```python
from build123d import *

# Parameters (mm, degrees)
F1_DEPTH = 27.4
F3_DEPTH = 10
F5_DEPTH = 88.2
F6_R     = 3.700156
F7_DEPTH = 27.768068


with BuildPart() as f1:
    # F0 (on Front) → F1 (new body, symmetric)
    with BuildSketch(Plane.XZ):
        Polygon((-10.816675, 0), (0, 0), (0, 27.767068), (-52.702516, 27.767068), (-52.702516, 10.254359), (-10.816675, 10.254359), align=None)
        Polygon((0, 27.767068), (0, 0), (10.816675, 0), (54.839961, 0), align=None)
    extrude(amount=F1_DEPTH, both=True)

    # F2 (on face) → F3 (cut)
    with BuildSketch(Plane.XZ.offset(27.4)):
        Polygon((10.816675, 22.290271), (10.816675, 0), (54.839961, 0), align=None)
    extrude(amount=-F3_DEPTH, mode=Mode.SUBTRACT)

    # F4 (on Right) → F5 (cut, symmetric)
    with BuildSketch(Plane.YZ):
        Polygon((-4.211452, 25.516083), (0, 25.516083), (4.211452, 25.516083), (4.211452, 28.770475), (-4.211452, 28.770475), align=None)
    extrude(amount=F5_DEPTH, both=True, mode=Mode.SUBTRACT)

    # F6 (on face) → F7 (cut, through all)
    with BuildSketch(Plane.XY.offset(27.767068)):
        with Locations((20, 17.4)):
            Circle(F6_R)
        with Locations((44.839961, 17.4)):
            Circle(F6_R)
        with Locations((44.839961, -7.4)):
            Circle(F6_R)
        with Locations((20, -7.4)):
            Circle(F6_R)
    extrude(amount=-F7_DEPTH, mode=Mode.SUBTRACT)


solid = f1.part
```
Geometry: final body of the model. Coordinates: model frame, mm. A direction names the side the tool comes from. Round coordinates to 2 decimals unless told otherwise and drop trailing zeros. Write each loop counter-clockwise with the first axis right and the second up, starting at its lowest first coordinate (ties: lowest second). Pieces come first, ordered by that corner, then holes.
Item 1: Section query B-B (y = -7.4). Return loops of the section in (x, z).
Item 2: Section query C-C (x = -28). Return loops of the section in (y, z), plus the area to 3 significant figures.
Item 3: Section query A-A (x = 20). Return loops of the section in (y, z), plus the area to 3 significant figures.
Item 4: Set-up query: faces 1 (the face through (-12, 27.4, 14)), 2 (the face through (-32, 0, 10.254)), 3 (the face through (10.817, -22, 11)), 4 (the face through (-24, 4.211, 27)). Return all of +Z, -Z, +X, -X, +Y, -Y with unobstructed straight access to the full face (end or side cutting, diameter ignored); none if empty.
Item 5: Section query D-D (y = 3). Return loops of the section in (x, z), plus the area to 3 significant figures.
Item 6: Material intervals for L1, parallel to X at y = -7, z = 4; L2, parallel to X at y = 17.4, z = 4; L3, parallel to Y at x = 22, z = 10.75, sorted ascending.
Item 7: Mould query, pull axis Y, two halves, no side actions, for faces 5 (the face through (-24, 0, 25.516)), 6 (the face through (-21, -27.4, 17)), 7 (the face through (-24, -4.211, 27)), 8 (the face through (27.8, 5.71, 13.69)). Classes: +Y half, -Y half, draft (parallel to the pull), parting line (faces both ways), or undercut.
Item 8: Pin query (flat end, axial travel): P1, Ø3, axis at y = 1.5, z = 7, coming from the -X side; P2, Ø8, axis at y = 16, z = 16, coming from the +X side; P3, Ø5, axis at y = -18, z = 10, coming from the +X side; P4, Ø6, axis at x = 20, y = -7.4, coming from the +Z side. Return the tip coordinate at first contact, or that it passes through.
Completed:
1. outline: (-52.7, 10.25) - (-10.82, 10.25) - (-10.82, 0) - (16.3, 0) - (16.3, 19.51) - (0, 27.77) - (-52.7, 27.77) - close; (23.7, 0) - (41.14, 0) - (41.14, 6.94) - (23.7, 15.77) - close; (48.54, 0) - (54.84, 0) - (48.54, 3.19) - close
2. outline: (-27.4, 10.25) - (27.4, 10.25) - (27.4, 27.77) - (4.21, 27.77) - (4.21, 25.52) - (-4.21, 25.52) - (-4.21, 27.77) - (-27.4, 27.77) - close
2. area: 941 mm2
3. outline: (-17.4, 0) - (-11.1, 0) - (-11.1, 17.64) - (-17.4, 17.64) - close; (-3.7, 0) - (13.7, 0) - (13.7, 17.64) - (-3.7, 17.64) - close; (21.1, 0) - (27.4, 0) - (27.4, 17.64) - (21.1, 17.64) - close
3. area: 529 mm2
4. face 1: +Z, -Z, +X, -X, +Y
4. face 2: -Z, -X, +Y, -Y
4. face 3: +Z, -Z, +X, -Y
4. face 4: +Z, +X, -X
5. outline: (-52.7, 10.25) - (-10.82, 10.25) - (-10.82, 0) - (54.84, 0) - (4.45, 25.52) - (-52.7, 25.52) - close
5. area: 1,670 mm2
6. L1: x = -10.82 to 16.32, 23.68 to 41.16
6. L2: x = -10.82 to 16.3, 23.7 to 41.14
6. L3: y = -17.4 to -10.51, -4.29 to 14.29, 20.51 to 27.4
7. face 5: undercut
7. face 6: -Y half
7. face 7: undercut
7. face 8: draft
8. P1: stops at x = -10.82
8. P2: stops at x = 31.14
8. P3: stops at x = 39.88
8. P4: passes through
